from build123d import *

# Parameters (mm, degrees)
SKETCH_W        = 46
SKETCH_H        = 120
SKETCH_R        = 2.7
PAD_DEPTH       = 12
SKETCH001_W     = 10
SKETCH001_H     = 120
POCKET_DEPTH    = 4
SKETCH002_W     = 46
SKETCH002_H     = 59
POCKET001_DEPTH = 1


with BuildPart() as part:
    # Sketch → Pad (new body)
    with BuildSketch(Plane.XY):
        with Locations((0, 60)):
            Rectangle(SKETCH_W, SKETCH_H)
        with Locations((-17, 7)):
            Circle(SKETCH_R, mode=Mode.SUBTRACT)
        with Locations((-17, 43)):
            Circle(SKETCH_R, mode=Mode.SUBTRACT)
        with Locations((17, 43)):
            Circle(SKETCH_R, mode=Mode.SUBTRACT)
        with Locations((17, 7)):
            Circle(SKETCH_R, mode=Mode.SUBTRACT)
        with Locations((-12, 115)):
            Circle(SKETCH_R, mode=Mode.SUBTRACT)
        with Locations((12, 115)):
            Circle(SKETCH_R, mode=Mode.SUBTRACT)
        with Locations((12, 75)):
            Circle(SKETCH_R, mode=Mode.SUBTRACT)
        with Locations((-12, 75)):
            Circle(SKETCH_R, mode=Mode.SUBTRACT)
    extrude(amount=PAD_DEPTH)

    # Sketch001 (on Face14 of Pad) → Pocket (cut)
    with BuildSketch(Plane.XY.offset(12)):
        with Locations((-0.080761, 60)):
            Rectangle(SKETCH001_W, SKETCH001_H)
    extrude(amount=-POCKET_DEPTH, mode=Mode.SUBTRACT)

    # Sketch002 (on Face2 of Pocket) → Pocket001 (cut)
    with BuildSketch(Plane(origin=(0, 0, 0), x_dir=(1, 0, 0), z_dir=(0, 0, -1))):
        with Locations((0, -90.5)):
            Rectangle(SKETCH002_W, SKETCH002_H)
    extrude(amount=-POCKET001_DEPTH, mode=Mode.SUBTRACT)


solid = part.part
Geometry check sheet. Reference: the model listing, model coordinates, mm. A direction names the side the tool comes from. Give positions to 0.01 mm unless a question says otherwise; leave off trailing zeros. Loops run counter-clockwise (first coordinate to the right, second up) from the corner with the lowest first, then second, coordinate; pieces in that order, holes last. Notation, with made-up numbers: M 2.5,42.25 L 31.5,42.25 A18 ccw 31.5,62.25 Z; hole C 85.5,36 d1. An arc over 180 degrees is marked long. Write each question's results on one line, items separated by ' | '.
1) Tool access check on faces 1 (the face through (-5.081, 59, 10)), 2 (the face through (0, 90, 1)), 3 (the face through (0, 0, 6)). Record the directions out of +Z, -Z, +X, -X, +Y, -Y that give a thin tool (end or side, any length) a straight path to the whole face; none if there is none.
Answers follow:
face 1: +Z, +Y, -Y | face 2: -Z, +X, -X, +Y | face 3: +Z, -Z, +X, -X, -Y
2) Section check D-D, the plane y = 94. Record the boundary of the cut face in (x, z), plus the area to 3 significant figures.
Answers follow:
outline: M -23,1 L 23,1 L 23,12 L 4.92,12 L 4.92,8 L -5.08,8 L -5.08,12 L -23,12 Z | area: 466 mm2
3) Release check for a two-part mould opening along Y. For faces 4 (the face through (19.575, 43.811, 5.916)), 5 (the face through (14, 61, 12)), 6 (the face through (0, 120, 6)) record: +Y half, -Y half, draft (parallel to the pull), parting line (faces both ways), or undercut.
Answers follow:
face 4: undercut | face 5: draft | face 6: +Y half
4) Section check B-B, the plane y = 7. Record the boundary of the cut face in (x, z), plus the area to 3 significant figures.
Answers follow:
outline: M -23,0 L -19.7,0 L -19.7,12 L -23,12 Z; M -14.3,0 L 14.3,0 L 14.3,12 L 4.92,12 L 4.92,8 L -5.08,8 L -5.08,12 L -14.3,12 Z; M 19.7,0 L 23,0 L 23,12 L 19.7,12 Z | area: 382 mm2
5) Section check A-A, the plane z = 10. Count the separate pieces of the cut face and the enclosed holes in it, plus the area to 3 significant figures.
Answers follow:
separate pieces: 2 | enclosed holes: 8 | area: 4,140 mm2
6) Gauge pin test, flat end, axial feed: pin 1 (1 mm diameter, centred on x = -15.5, y = 86.5, fed in from -Z). Record the tip position at first contact, or that the pin passes through.
Answers follow:
pin 1: z = 1
7) Thickness scan on line 1 (X direction, y = 75, z = 7.5); line 2 (Y direction, x = -12, z = 8.25); line 3 (Y direction, x = -13.5, z = 2) (3 decimals). Record the ranges inside material, lowest first.
Answers follow:
line 1: -23 to -14.7, -9.3 to 9.3, 14.7 to 23 | line 2: 0 to 72.3, 77.7 to 112.3, 117.7 to 120 | line 3: 0 to 72.755, 77.245 to 112.755, 117.245 to 120
8) Section check C-C, the plane x = -17. Record the boundary of the cut face in (y, z), plus the area to 3 significant figures.
Answers follow:
outline: M 0,0 L 4.3,0 L 4.3,12 L 0,12 Z; M 9.7,0 L 40.3,0 L 40.3,12 L 9.7,12 Z; M 45.7,0 L 61,0 L 61,1 L 120,1 L 120,12 L 45.7,12 Z | area: 1,250 mm2
